Design review of the part built by this model. Coordinates are the model's own, in mm. Face numbers are marked on the shaded views. Give positions to 0.01 mm unless a question says otherwise; leave off trailing zeros. Order: outer loops, then holes, each group sorted by start corner. A loop starts at its lowest first (then second) coordinate and runs counter-clockwise, first axis right, second up. Notation, with made-up numbers: (46, 1.5) -> (79, 1.5) arc R14 cw to (79, 13.5) -> close; hole circle Ø10 at (48, -21). An arc over 180 degrees is marked (long way). Use a Markdown table: item, result. Add a question column.
```python
from build123d import *

# Parameters (mm, degrees)
SKETCH1_W           = 200
SKETCH1_H           = 100
BOSS_EXTRUDE1_DEPTH = 3
SKETCH2_W           = 5
SKETCH2_H           = 100
BOSS_EXTRUDE2_DEPTH = 15
CUT_EXTRUDE1_REACH  = 208.94
SKETCH3_R           = 2
LPATTERN1_COUNT     = 2
LPATTERN1_PITCH     = 80
CUT_EXTRUDE2_REACH  = 114.805
SKETCH4_R           = 2
LPATTERN2_COUNT     = 2
LPATTERN2_PITCH     = 80
SKETCH5_W           = 160
SKETCH5_H           = 3
BOSS_EXTRUDE3_DEPTH = 15
CUT_EXTRUDE3_REACH  = 144.562
SKETCH6_R           = 1.5


with BuildPart() as part:
    # Sketch1 → Boss-Extrude1 (new body)
    with BuildSketch(Plane(origin=(0, 0, 0), x_dir=(1, 0, 0), z_dir=(0, 1, 0))):
        Rectangle(SKETCH1_W, SKETCH1_H)
    extrude(amount=BOSS_EXTRUDE1_DEPTH)

    # Sketch2 → Boss-Extrude2 (add)
    with BuildSketch(Plane(origin=(0, 3, 0), x_dir=(1, 0, 0), z_dir=(0, 1, 0))):
        with Locations((-97.5, 0)):
            Rectangle(SKETCH2_W, SKETCH2_H)
    extrude(amount=BOSS_EXTRUDE2_DEPTH)

    # Sketch3 → Cut-Extrude1 (cut, up to next)
    with BuildSketch(Plane.ZY.offset(100), mode=Mode.PRIVATE) as cut_extrude1_sk1:
        with Locations((40, 10)):
            Circle(SKETCH3_R)
    cut_extrude1_tool1 = extrude(cut_extrude1_sk1.sketch, amount=-CUT_EXTRUDE1_REACH, mode=Mode.PRIVATE) & part.part
    cut_extrude1 = cut_extrude1_tool1.solids().sort_by_distance((-100, 10, 40))[0]
    add(cut_extrude1, mode=Mode.SUBTRACT)

    # LPattern1: Cut-Extrude1 ×2
    with Locations(*[(0, 0, -i * LPATTERN1_PITCH) for i in range(1, LPATTERN1_COUNT)]):
        add(cut_extrude1, mode=Mode.SUBTRACT)

    # Sketch4 → Cut-Extrude2 (cut, up to next)
    with BuildSketch(Plane(origin=(0, 3, 0), x_dir=(1, 0, 0), z_dir=(0, 1, 0)), mode=Mode.PRIVATE) as cut_extrude2_sk1:
        with Locations(Location((95, 40, 0), (0, 0, 270))):
            Circle(SKETCH4_R)
    cut_extrude2_tool1 = extrude(cut_extrude2_sk1.sketch, amount=-CUT_EXTRUDE2_REACH, mode=Mode.PRIVATE) & part.part
    cut_extrude2 = cut_extrude2_tool1.solids().sort_by_distance((95, 3, -40))[0]
    add(cut_extrude2, mode=Mode.SUBTRACT)

    # LPattern2: Cut-Extrude2 ×2
    with Locations(*[(0, 0, i * LPATTERN2_PITCH) for i in range(1, LPATTERN2_COUNT)]):
        add(cut_extrude2, mode=Mode.SUBTRACT)

    # Sketch5 → Boss-Extrude3 (add)
    with BuildSketch(Plane(origin=(0, 3, 0), x_dir=(1, 0, 0), z_dir=(0, 1, 0))):
        with Locations((-15, 48.5)):
            Rectangle(SKETCH5_W, SKETCH5_H)
    extrude(amount=BOSS_EXTRUDE3_DEPTH)

    # Sketch6 → Cut-Extrude3 (cut, up to next)
    with BuildSketch(Plane(origin=(0, 0, -50), x_dir=(-1, 0, 0), z_dir=(0, 0, -1)), mode=Mode.PRIVATE) as cut_extrude3_sk1:
        with Locations((85, 10)):
            Circle(SKETCH6_R)
    cut_extrude3_tool1 = extrude(cut_extrude3_sk1.sketch, amount=-CUT_EXTRUDE3_REACH, mode=Mode.PRIVATE) & part.part
    # Sketch6 → Cut-Extrude3 (cut, up to next)
    with BuildSketch(Plane(origin=(0, 0, -50), x_dir=(-1, 0, 0), z_dir=(0, 0, -1)), mode=Mode.PRIVATE) as cut_extrude3_sk2:
        with Locations((17.5, 10)):
            Circle(SKETCH6_R)
    cut_extrude3_tool2 = extrude(cut_extrude3_sk2.sketch, amount=-CUT_EXTRUDE3_REACH, mode=Mode.PRIVATE) & part.part
    # Sketch6 → Cut-Extrude3 (cut, up to next)
    with BuildSketch(Plane(origin=(0, 0, -50), x_dir=(-1, 0, 0), z_dir=(0, 0, -1)), mode=Mode.PRIVATE) as cut_extrude3_sk3:
        with Locations((-50, 10)):
            Circle(SKETCH6_R)
    cut_extrude3_tool3 = extrude(cut_extrude3_sk3.sketch, amount=-CUT_EXTRUDE3_REACH, mode=Mode.PRIVATE) & part.part
    add(cut_extrude3_tool1.solids().sort_by_distance((-85, 10, -50))[0], mode=Mode.SUBTRACT)
    add(cut_extrude3_tool2.solids().sort_by_distance((-17.5, 10, -50))[0], mode=Mode.SUBTRACT)
    add(cut_extrude3_tool3.solids().sort_by_distance((50, 10, -50))[0], mode=Mode.SUBTRACT)


solid = part.part
```
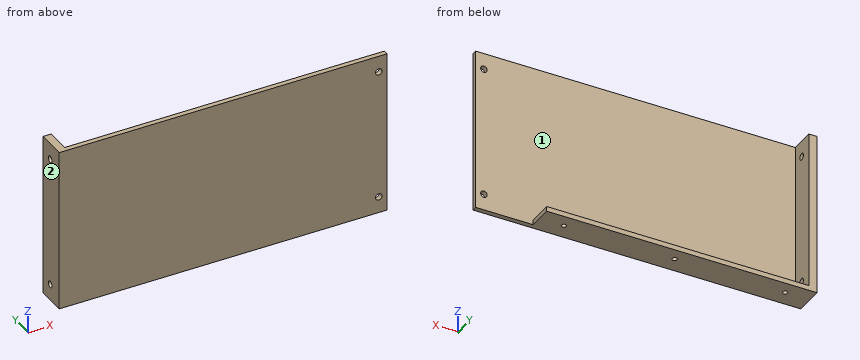
1) Insertion check: pin 1 (1 mm diameter, centred on y = 6.5, z = 13.5, fed in from +X); pin 2 (2.5 mm diameter, centred on y = 10, z = -48, fed in from +X); pin 3 (4 mm diameter, centred on x = -17.5, y = 10, fed in from +Z). Each pin has a flat end and moves straight along its axis. Give the tip position at first contact, or say it passes through.
2) Add section B-B (z = 40). Give the boundary of the cut face in (x, y), then the cut area to 3 significant figures.
3) For L1, parallel to Y at x = 44.5, z = 9; L2, parallel to Z at x = -39, y = 9.5; L3, parallel to X at y = 12.5, z = -41, list the stretches that pass through material, from the lowest coordinate up. Write a range as [from, to].
4) The part is to be moulded in two halves that separate along X. For the marked faces 1 and 2, say which applies: +X half, -X half, draft (parallel to the pull), parting line (faces both ways), or undercut.
5) Add section C-C (z = 26.5). Give the boundary of the cut face in (x, y), then the cut area to 3 significant figures.
6) Add section A-A (x = 95). Give the boundary of the cut face in (y, z).
7) Add section D-D (x = 23). Give the boundary of the cut face in (y, z).
Worked answers:
| question | item | result |
|---|---|---|
| 1 | pin 1 | x = -95 |
| 1 | pin 2 | x = 65 |
| 1 | pin 3 | z = -47 |
| 2 | outline | (-100, 0) -> (93, 0) -> (93, 3) -> (-95, 3) -> (-95, 8) -> (-100, 8) -> close; (-100, 12) -> (-95, 12) -> (-95, 18) -> (-100, 18) -> close; (97, 0) -> (100, 0) -> (100, 3) -> (97, 3) -> close |
| 2 | area | 643 mm^2 |
| 3 | L1 | [0, 3] |
| 3 | L2 | [-50, -47] |
| 3 | L3 | [-100, -95] |
| 4 | face 1 | draft |
| 4 | face 2 | -X half |
| 5 | outline | (-100, 0) -> (100, 0) -> (100, 3) -> (-95, 3) -> (-95, 18) -> (-100, 18) -> close |
| 5 | area | 675 mm^2 |
| 6 | outline | (0, -50) -> (3, -50) -> (3, -42) -> (0, -42) -> close; (0, -38) -> (3, -38) -> (3, 38) -> (0, 38) -> close; (0, 42) -> (3, 42) -> (3, 50) -> (0, 50) -> close |
| 7 | outline | (0, -50) -> (18, -50) -> (18, -47) -> (3, -47) -> (3, 50) -> (0, 50) -> close |
